Check sheet for the modelled part. Datum: model origin and axes. Units: mm. A direction names the side the tool comes from. Round coordinates to 2 decimals unless told otherwise and drop trailing zeros. Write each loop counter-clockwise with the first axis right and the second up, starting at its lowest first coordinate (ties: lowest second). Pieces come first, ordered by that corner, then holes. Notation, with made-up numbers: M 19,39.5 L 35,39.5 A24 cw 35,52.5 Z; hole C -6.75,-19 d9. An arc over 180 degrees is marked long. Put each result on its own line as item: value.
Autodesk Inventor part; units mm, degrees
ref_plane "YZ Plane" through (0, 0, 0) normal (1, 0, 0) x (0, 1, 0)
ref_plane "XZ Plane" through (0, 0, 0) normal (0, 1, 0) x (-1, 0, 0)
ref_plane "XY Plane" through (0, 0, 0) normal (0, 0, 1) x (1, 0, 0)
sketch "Sketch1" plane through (0, 0, 0) normal (0, 0, 1) x (1, 0, 0)
  line L0 (0, 0) -> (102, 0)
  line L1 (102, 0) -> (102, 1.7)
  line L2 (102, 1.7) -> (0, 1.7)
  line L3 (0, 1.7) -> (0, 0)
  dimension "d0" = 102
  dimension "d1" = 1.7
extrude "Extrusion1" add sketch "Sketch1" along normal blind 53.3
sketch "Sketch3" plane through (0, 1.7, 53.3) normal (0, 1, 0) x (1, 0, 0)
  line L0 (102, 53.3) -> (0, 53.3)
  line L1 (0, 53.3) -> (0, 0)
  line L2 (0, 0) -> (102, 0)
  line L3 (9.75, 44.2) -> (-6.65, 44.2)
  line L4 (-6.65, 44.2) -> (-6.65, 32)
  line L5 (-6.65, 32) -> (9.75, 32)
  line L6 (9.75, 32) -> (9.75, 44.2)
  line L7 (12.3, 12.4) -> (-1.7, 12.4)
  line L8 (-1.7, 12.4) -> (-1.7, 3.6)
  line L9 (-1.7, 3.6) -> (12.3, 3.6)
  line L10 (12.3, 3.6) -> (12.3, 12.4)
  line L11 (102, 0) -> (0, 0)
  line L12 (99, 0) -> (99, 1.4)
  line L13 (99, 1.4) -> (102, 4)
  line L14 (102, 4) -> (102, 39.12)
  line L15 (102, 53.3) -> (102, 0)
  line L16 (102, 39.12) -> (98.6, 41.3)
  line L17 (98.6, 41.3) -> (98.6, 50.3)
  line L18 (98.6, 50.3) -> (95.6, 53.3)
  line L19 (0, 53.3) -> (102, 53.3)
  circle A0 centre (96.75, 2.55) radius 1.65
  circle A1 centre (90.05, 50.75) radius 1.65
  circle A2 centre (66.35, 35.45) radius 1.65
  circle A3 centre (66.35, 7.65) radius 1.65
  circle A4 centre (15.25, 50.75) radius 1.65
  circle A5 centre (14.25, 2.55) radius 1.65
  line L20 (88.15, 49.5) -> (17.15, 49.5)
  line L21 (17.15, 49.5) -> (17.15, 52)
  line L22 (17.15, 52) -> (88.15, 52)
  line L23 (88.15, 52) -> (88.15, 49.5)
  line L24 (93.3, 1.3) -> (26.8, 1.3)
  line L25 (26.8, 1.3) -> (26.8, 3.8)
  line L26 (26.8, 3.8) -> (93.3, 3.8)
  line L27 (93.3, 3.8) -> (93.3, 1.3)
  line L28 (97.65, 52.2) -> (92.65, 52.2)
  line L29 (92.65, 52.2) -> (92.65, 5.8)
  line L30 (92.65, 5.8) -> (97.65, 5.8)
  line L31 (97.65, 5.8) -> (97.65, 52.2)
  dimension "d23" = 9.1
  dimension "d24" = 9.75
  dimension "d25" = 16.4
  dimension "d26" = 12.2
  dimension "d27" = 8.8
  dimension "d28" = 14
  dimension "d29" = 12.4
  dimension "d30" = 1.7
  dimension "d44" = 3
  dimension "d45" = 3.4
  dimension "d46" = 3
  dimension "d47" = 3
  dimension "d48" = 1.4
  dimension "d49" = 4
  dimension "d50" = 35.12
  dimension "d51" = 12
  dimension "d52" = 3.3
  dimension "d53" = 3.3
  dimension "d54" = 3.3
  dimension "d55" = 3.3
  dimension "d56" = 3.3
  dimension "d57" = 3.3
  dimension "d58" = 0.9
  dimension "d59" = 3.6
  dimension "d60" = 6.9
  dimension "d61" = 0.9
  dimension "d62" = 0.9
  dimension "d63" = 0.9
  dimension "d64" = 13.6
  dimension "d66" = 12.6
  dimension "d67" = 34
  dimension "d69" = 34
  dimension "d70" = 6
  dimension "d71" = 16.2
  dimension "d72" = 71
  dimension "d73" = 0.25
  dimension "d74" = 2.5
  dimension "d75" = 1.25
  dimension "d76" = 66.5
  dimension "d77" = 2.5
  dimension "d78" = 1.25
  dimension "d79" = 1.8
  dimension "d80" = 5
  dimension "d81" = 46.4
  dimension "d82" = 1.1
  dimension "d83" = 0.95
extrude "Extrusion3" add sketch "Sketch3" along normal blind 10.8 contours L3 L6 L5 L1 | L1 L5 L4 L3 | L7 L10 L9 L1 | L1 L9 L8 L7
extrude "Extrusion9" cut sketch "Sketch3" against normal blind 10 contours L15 L16 L17 L18 L31 L28 L0 | L28 L31 L18 | L15 L2 L12 L13 | A0 | A1 | A2 | A3 | A4 | A5
extrude "Extrusion10" add sketch "Sketch3" along normal blind 8.7 contours L28 L31 L18 | L18 L31 L30 L29 L28 | L20 L21 L22 L23 | L24 L25 L26 L27
sketch "Sketch7" plane through (0, 0, 0) normal (0, -1, 0) x (1, 0, 0)
  line L0 (26.8, 52) -> (26.8, 49.5)
  line L1 (93.3, 52) -> (26.8, 52)
  line L2 (93.3, 49.5) -> (93.3, 52)
  line L3 (26.8, 49.5) -> (93.3, 49.5)
  line L4 (17.15, 3.8) -> (17.15, 1.3)
  line L5 (88.15, 3.8) -> (17.15, 3.8)
  line L6 (88.15, 1.3) -> (88.15, 3.8)
  line L7 (17.15, 1.3) -> (88.15, 1.3)
  line L8 (97.65, 1.1) -> (97.65, 47.5)
  line L9 (92.65, 1.1) -> (97.65, 1.1)
  line L10 (92.65, 47.5) -> (92.65, 1.1)
  line L11 (97.65, 47.5) -> (92.65, 47.5)
  line L12 (87.5288, 2.0107) -> (17.9769, 2.0107)
  line L13 (17.9769, 2.0107) -> (17.9769, 3.0107)
  line L14 (17.9769, 3.0107) -> (87.5288, 3.0107)
  line L15 (87.5288, 3.0107) -> (87.5288, 2.0107)
  line L16 (92.4851, 50.2518) -> (27.6531, 50.2518)
  line L17 (27.6531, 50.2518) -> (27.6531, 51.2518)
  line L18 (27.6531, 51.2518) -> (92.4851, 51.2518)
  line L19 (92.4851, 51.2518) -> (92.4851, 50.2518)
  line L20 (96.9467, 2.0107) -> (95.9467, 2.0107)
  line L21 (95.9467, 2.0107) -> (95.9467, 46.8913)
  line L22 (95.9467, 46.8913) -> (96.9467, 46.8913)
  line L23 (96.9467, 46.8913) -> (96.9467, 2.0107)
  line L24 (93.4467, 46.8913) -> (94.4467, 46.8913)
  line L25 (94.4467, 46.8913) -> (94.4467, 2.0107)
  line L26 (94.4467, 2.0107) -> (93.4467, 2.0107)
  line L27 (93.4467, 2.0107) -> (93.4467, 46.8913)
  line L28 (12.3, 40.9) -> (12.3, 49.7)
  line L29 (-1.7, 40.9) -> (12.3, 40.9)
  line L30 (-1.7, 49.7) -> (-1.7, 40.9)
  line L31 (12.3, 49.7) -> (-1.7, 49.7)
  line L32 (9.75, 9.1) -> (9.75, 21.3)
  line L33 (-6.65, 9.1) -> (9.75, 9.1)
  line L34 (-6.65, 21.3) -> (-6.65, 9.1)
  line L35 (9.75, 21.3) -> (-6.65, 21.3)
  line L36 (0, 9.1) -> (9.75, 9.1)
  line L37 (6.6731, 6.8776) -> (3.1632, 6.8776)
  line L38 (3.1632, 6.8776) -> (3.1632, 9.1)
  line L39 (3.1632, 9.1) -> (6.6731, 9.1)
  line L40 (6.6731, 9.1) -> (6.6731, 6.8776)
  line L41 (9.75, 21.3) -> (0, 21.3)
  line L42 (6.6731, 21.3) -> (3.1632, 21.3)
  line L43 (3.1632, 21.3) -> (3.1632, 24.3)
  line L44 (3.1632, 24.3) -> (6.6731, 24.3)
  line L45 (6.6731, 24.3) -> (6.6731, 21.3)
  line L46 (9.75, 44) -> (2.1298, 44)
  line L47 (2.1298, 44) -> (2.1298, 51.9)
  line L48 (2.1298, 51.9) -> (9.75, 51.9)
  line L49 (9.75, 51.9) -> (9.75, 44)
  dimension "d110" = 1
  dimension "d111" = 1
  dimension "d112" = 1
  dimension "d113" = 1.5
  dimension "d114" = 1
extrude "Extrusion12" add sketch "Sketch7" along normal blind 1.3 contours L12 L13 L14 L15 | L16 L17 L18 L19 | L20 L21 L22 L23 | L24 L25 L26 L27
extrude "Extrusion13" add sketch "Sketch7" along normal blind 2.5 contours L49 L46 L47 L31 | L31 L47 L48 L49 | L40 L37 L38 L33 | L35 L43 L44 L45
properties part number "Arduino"
1. Release check for a two-part mould opening along X. For faces 4 (the flat face through (61, 6, 52)), 5 (the flat face through (93.3, 6, 51)), 6 (the flat face through (9.75, -1, 48)), 7 (the flat face through (50, 0, 26)) record: +X half, -X half, draft (parallel to the pull), parting line (faces both ways), or undercut.
Computed values:
face 4: draft
face 5: +X half
face 6: undercut
face 7: undercut
2. Access from +Z, -Z, +X, -X, +Y, -Y to the whole of each face (thin tool, end or side, straight path). Record for faces 1 (the flat face through (-3, 1.7, 15)), 2 (the flat face through (12.3, 7, 45)), 3 (the flat face through (1, 7, 21.3)).
Computed values:
face 1: +Z, -Z, -X, -Y
face 2: +Z, -Z, +Y
face 3: -X, +Y
3. Cross-section at C-C (z = 17.85). Enter the section's corners in (x, y), then the cut area to 3 significant figures.
Computed values:
outline: M -6.65,1.7 L 0,1.7 L 0,0 L 64.7,0 L 64.7,1.7 L 9.75,1.7 L 9.75,12.5 L -6.65,12.5 Z; M 68,0 L 93.45,0 L 93.45,-1.3 L 94.45,-1.3 L 94.45,0 L 95.95,0 L 95.95,-1.3 L 96.95,-1.3 L 96.95,0 L 102,0 L 102,1.7 L 97.65,1.7 L 97.65,10.4 L 92.65,10.4 L 92.65,1.7 L 68,1.7 Z
area: 391 mm2
4. Depth check by flat-ended pin: pin 1 Ø6 at (x, y) = (73, 11) entering from +Z; pin 2 Ø4.5 at (x, z) = (66.35, 17.85) entering from +Y; pin 3 Ø0.6 at (y, z) = (-1, 30.5) entering from +X. Enter the tip coordinate at first touch or a pass-through.
Computed values:
pin 1: stops at z = 52
pin 2: stops at y = 1.7
pin 3: stops at x = 96.95
5. Cross-section at D-D (x = 66.35). Enter the section's corners in (y, z), then the cut area to 3 significant figures.
Computed values:
outline: M -1.3,2.01 L 0,2.01 L 0,0 L 1.7,0 L 1.7,1.3 L 10.4,1.3 L 10.4,3.8 L 1.7,3.8 L 1.7,16.2 L 0,16.2 L 0,3.01 L -1.3,3.01 Z; M -1.3,50.25 L 0,50.25 L 0,47.3 L 1.7,47.3 L 1.7,49.5 L 10.4,49.5 L 10.4,52 L 1.7,52 L 1.7,53.3 L 0,53.3 L 0,51.25 L -1.3,51.25 Z; M 0,19.5 L 1.7,19.5 L 1.7,44 L 0,44 Z
area: 125 mm2
6. Scan lines: probe 1 along X at (y, z) = (0.85, 17.85); probe 2 along Z at (x, y) = (87, 10.25); probe 3 along X at (y, z) = (6, 10.5). Record each from-to range of solid material in increasing order.
Computed values:
probe 1: x = 0 to 64.7, 68 to 102
probe 2: z = 1.3 to 3.8, 49.5 to 52
probe 3: x = -6.65 to 9.75, 92.65 to 97.65
7. Cross-section at B-B (y = 8.25). Enter the section's corners in (x, z).
Computed values:
outline: M -6.65,9.1 L 9.75,9.1 L 9.75,21.3 L -6.65,21.3 Z; M -1.7,40.9 L 12.3,40.9 L 12.3,49.7 L -1.7,49.7 Z; M 17.15,1.3 L 88.15,1.3 L 88.15,3.8 L 17.15,3.8 Z; M 26.8,49.5 L 93.3,49.5 L 93.3,52 L 26.8,52 Z; M 92.65,1.1 L 97.65,1.1 L 97.65,47.5 L 92.65,47.5 Z
8. Cross-section at A-A (x = 90.05). Enter the section's corners in (y, z), then the cut area to 3 significant figures.
Computed values:
outline: M -1.3,50.25 L 0,50.25 L 0,4.2 L 1.7,4.2 L 1.7,49.5 L 10.4,49.5 L 10.4,52 L 1.7,52 L 1.7,53.3 L 0,53.3 L 0,51.25 L -1.3,51.25 Z; M 0,0 L 1.7,0 L 1.7,0.9 L 0,0.9 Z
area: 108 mm2
